```python
from build123d import *

# Parameters (mm, degrees)
SKETCH2_R            = 39.37
SKETCH2_R_2          = 38.1
BASE_CYLINDER_DEPTH  = 292.1
SKETCH3_R            = 63.5
SKETCH3_R_2          = 38.1
AFT_FLANGE_DEPTH     = 12.7
SKETCH4_R            = 63.5
SKETCH4_R_2          = 38.1
FORWARD_FLANGE_DEPTH = 12.7


with BuildPart() as part:
    # Sketch2 → Base Cylinder (new body)
    with BuildSketch(Plane(origin=(0, 0, 0), x_dir=(1, 0, 0), z_dir=(0, 1, 0))):
        Circle(SKETCH2_R)
        Circle(SKETCH2_R_2, mode=Mode.SUBTRACT)
    extrude(amount=BASE_CYLINDER_DEPTH)

    # Sketch3 → Aft Flange (add)
    with BuildSketch(Plane.XZ):
        Circle(SKETCH3_R)
        Circle(SKETCH3_R_2, mode=Mode.SUBTRACT)
    extrude(amount=-AFT_FLANGE_DEPTH)

    # Sketch4 → Forward Flange (add)
    with BuildSketch(Plane(origin=(0, 292.1, 0), x_dir=(1, 0, 0), z_dir=(0, 1, 0))):
        Circle(SKETCH4_R)
        Circle(SKETCH4_R_2, mode=Mode.SUBTRACT)
    extrude(amount=-FORWARD_FLANGE_DEPTH)


solid = part.part
```
Can you work these out from the model? Positions are in its coordinate system, mm. A direction names the side the tool comes from. Coordinates: 2 decimals unless noted, no trailing zeros. Loops run counter-clockwise (first coordinate to the right, second up) from the corner with the lowest first, then second, coordinate; pieces in that order, holes last. Notation, with made-up numbers: M 36.5,43.25 L 91.5,43.25 A12 cw 91.5,59.25 Z; hole C 29,78.5 d4. An arc over 180 degrees is marked long. Put each result on its own line as item: value. Start each with the question number.
(1) We'd pull the mould along Z, two halves only. Please class faces 3 (the face through (27, 279.4, -29)), 4 (the face through (-31.24, 144.18, 23.96)), 5 (the face through (-30.235, 144.005, 23.183)): +Z half, -Z half, draft (parallel to the pull), parting line (faces both ways), or undercut.
(2) Imagine slicing it at C-C on y = 240. List the corners of the cut face in (x, z) for me, and give its area (3 significant figures).
(3) Imagine slicing it at D-D on z = -52. List the corners of the cut face in (x, y) for me, and give its area (3 significant figures).
(4) Which directions (+Z, -Z, +X, -X, +Y, -Y) give clear straight access to the entire face, cutting with the end or side of a thin tool? Please do faces 1 (the face through (27.3, 292.1, 27.3)), 2 (the face through (27, 12.7, 29)).
(5) I need wall thicknesses on probe 1 along Y at (x, z) = (-50, -15.5); probe 2 along Z at (x, y) = (0, 106); probe 3 along X at (y, z) = (110, 2.5). Which ranges of each line are inside material? Lowest first, please.
(6) Will these pins go through, and if not, where does the flat tip stop? pin 1 Ø1 at (x, y) = (4.5, 260) entering from +Z; pin 2 Ø3 at (y, z) = (169.5, 2.5) entering from -X; pin 3 Ø10 at (y, z) = (192, 4.5) entering from +X.
(7) Imagine slicing it at B-B on z = 0. List the corners of the cut face in (x, y) for me, and give its area (3 significant figures).
(8) Imagine slicing it at A-A on x = 0. List the corners of the cut face in (y, z) for me.
Worked answers:
1. face 3: draft
1. face 4: parting line
1. face 5: undercut
2. outline: C 0,0 d78.74; hole C 0,0 d76.2
2. area: 309 mm2
3. outline: M -36.45,0 L 36.45,0 L 36.45,12.7 L -36.45,12.7 Z; M -36.45,279.4 L 36.45,279.4 L 36.45,292.1 L -36.45,292.1 Z
3. area: 1,850 mm2
4. face 1: +Z, -Z, +X, -X, +Y
4. face 2: none
5. probe 1: y = 0 to 12.7, 279.4 to 292.1
5. probe 2: z = -39.37 to -38.1, 38.1 to 39.37
5. probe 3: x = -39.29 to -38.02, 38.02 to 39.29
6. pin 1: stops at z = 39.17
6. pin 2: stops at x = -39.36
6. pin 3: stops at x = 39.37
7. outline: M -63.5,0 L -38.1,0 L -38.1,292.1 L -63.5,292.1 L -63.5,279.4 L -39.37,279.4 L -39.37,12.7 L -63.5,12.7 Z; M 38.1,0 L 63.5,0 L 63.5,12.7 L 39.37,12.7 L 39.37,279.4 L 63.5,279.4 L 63.5,292.1 L 38.1,292.1 Z
7. area: 1,970 mm2
8. outline: M 0,-63.5 L 12.7,-63.5 L 12.7,-39.37 L 279.4,-39.37 L 279.4,-63.5 L 292.1,-63.5 L 292.1,-38.1 L 0,-38.1 Z; M 0,38.1 L 292.1,38.1 L 292.1,63.5 L 279.4,63.5 L 279.4,39.37 L 12.7,39.37 L 12.7,63.5 L 0,63.5 Z
